Design review of the part built by this model. Coordinates are the model's own, in mm. Round coordinates to 2 decimals unless told otherwise and drop trailing zeros. Order: outer loops, then holes, each group sorted by start corner. A loop starts at its lowest first (then second) coordinate and runs counter-clockwise, first axis right, second up. Notation, with made-up numbers: (40, -32) - (73, -32) arc R24 ccw to (73, 4) - close; hole circle Ø1 at (40.25, 17.5). An arc over 180 degrees is marked (long way). Write item = value, one per line.
Autodesk Inventor part; units mm, degrees
ref_plane "YZ Plane" through (0, 0, 0) normal (1, 0, 0) x (0, 1, 0)
ref_plane "XZ Plane" through (0, 0, 0) normal (0, 1, 0) x (-1, 0, 0)
ref_plane "XY Plane" through (0, 0, 0) normal (0, 0, 1) x (1, 0, 0)
sketch "Szkic1" plane through (0, 0, 0) normal (0, 0, 1) x (1, 0, 0)
  line L0 (75.0555, 130) -> (150.1111, 0)
  line L1 (150.1111, 0) -> (75.0555, -130)
  line L2 (75.0555, -130) -> (-75.0555, -130)
  line L3 (-75.0555, -130) -> (-150.1111, 0)
  line L4 (-150.1111, 0) -> (-75.0555, 130)
  line L5 (-75.0555, 130) -> (75.0555, 130)
  point P0 (0, 0)
  point P1 (0, 0)
  dimension "d0" = 130
extrude "Płyta1" add sketch "Szkic1" along normal blind 0.8
ref_plane "Płaszczyzna konstrukcyjna2" through (112.5833, 65, 0.8) normal (-0.5, 0.8660254, 0) x (0, 0, -1)
ref_plane "Płaszczyzna konstrukcyjna3" through (-112.5833, 65, 0) normal (0.5, 0.8660254, 0) x (0, 0, 1)
sketch "Szkic22" plane through (0, 0, 0) normal (0, 0, -1) x (-1, 0, 0)
  circle A0 centre (-120, 0) radius 1.5
  point P0 (0, 0)
  point P1 (-60, -103.923)
  point P2 (60, -103.923)
  point P3 (120, 0)
  point P4 (60, 103.923)
  point P5 (-60, 103.923)
  dimension "d132" = 360
hole "Otwór7" at (120, 0, 0) at (60, -103.923, 0) at (-60, -103.923, 0) at (-120, 0, 0) at (-60, 103.923, 0) at (60, 103.923, 0) direction (0, 0, 1) diameter 3 depth 0.8 tip angle 118
sketch "Szkic23" plane through (0, 0, 0) normal (0, 0, -1) x (-1, 0, 0)
  circle A0 centre (-96.057, -71.6244) radius 2
  circle A1 centre (-110.057, -47.3756) radius 2
  line L0 (-106.6109, -41.3446) -> (-89.1109, -71.6554)
  line L1 (-89.1109, -71.6554) -> (-99.5032, -77.6554)
  line L2 (-117.0032, -47.3446) -> (-99.5032, -77.6554)
  line L3 (-106.6109, -41.3446) -> (-117.0032, -47.3446)
  circle A2 centre (110.057, -47.3756) radius 2
  circle A3 centre (96.057, -71.6244) radius 2
  line L4 (89.1109, -71.6554) -> (106.6109, -41.3446)
  line L5 (106.6109, -41.3446) -> (117.0032, -47.3446)
  line L6 (99.5032, -77.6554) -> (117.0032, -47.3446)
  line L7 (89.1109, -71.6554) -> (99.5032, -77.6554)
  circle A4 centre (-14, 119) radius 2
  circle A5 centre (14, 119) radius 2
  line L8 (17.5, 113) -> (-17.5, 113)
  line L9 (-17.5, 113) -> (-17.5, 125)
  line L10 (17.5, 125) -> (-17.5, 125)
  line L11 (17.5, 113) -> (17.5, 125)
  point P0 (0, 0)
hole "Otwór8" at (-96.057, -71.6244, 0) at (-110.057, -47.3756, 0) at (-14, 119, 0) at (14, 119, 0) at (110.057, -47.3756, 0) at (96.057, -71.6244, 0) direction (0, 0, 1) diameter 4 depth 0.8 tip angle 118
equation "\"d139\" = Grubość"
equation "\"d146\" = Grubość"
equation "\"PromieńGięcia\" = Grubość"
equation "\"SzerokośćGięciaPodcięcia\" = Grubość"
equation "\"GłębokośćGięciaPodcięcia\" = 0.5 * Grubość"
equation "\"RozmiarPodcięciaNarożnika\" = 4 * Grubość"
equation "\"MinimalnaPozostałość\" = 2 * Grubość"
equation "\"PromieńPrzejścia\" = PromieńGięcia"
equation "\"Rozmiar_promienia_Jacobiego\" = Grubość"
equation "\"Wielk_odstępu\" = Grubość"
equation "\"d1\" = PromieńGięcia"
properties part number "base_bottom"
Item 1: For line 1 along X through (y, z) = (95, 0.2); line 2 along X through (y, z) = (74.5, 0.7); line 3 along Y through (x, z) = (113, 0.7), list the stretches that pass through material, from the lowest coordinate up. Write a range as [from, to].
Data:
line_1 = [-95.26, 95.26]
line_2 = [-107.1, 107.1]
line_3 = [-64.28, 64.28]
Item 2: Take a section at C-C, the plane x = -88. State the section outline as (y, z) points.
Data:
outline = (-107.58, 0) - (107.58, 0) - (107.58, 0.8) - (-107.58, 0.8) - close
Item 3: Take a section at B-B, the plane y = -9.5. State the section outline as (x, z) points.
Data:
outline = (-144.63, 0) - (144.63, 0) - (144.63, 0.8) - (-144.63, 0.8) - close
Item 4: Insertion check: P1, Ø2.5, axis at x = 96.06, y = -71.62, coming from the +Z side. The pin has a flat end and moves straight along its axis. Give the tip position at first contact, or say it passes through.
Data:
P1 = through
Item 5: Take a section at A-A, the plane z = 0.6. Count the separate pieces of the cut face and the enclosed holes in it, and give its area (3 significant figures).
Data:
separate_pieces = 1
enclosed_holes = 12
area = 58,400 mm2
